Work out the finished part from the listing and answer in its coordinate system (mm). Face numbers are marked on the shaded views. A direction names the side the tool comes from. Coordinates: 2 decimals unless noted, no trailing zeros. Order: outer loops, then holes, each group sorted by start corner. A loop starts at its lowest first (then second) coordinate and runs counter-clockwise, first axis right, second up.
1. A tool of negligible diameter and unlimited length cuts with its end or side. For the marked faces 5, 6 and 7, from which of +Z, -Z, +X, -X, +Y, -Y can it reach the whole face along a straight path? Write none if from no direction.
2. The part is cut by section C-C, the plane x = -49. Give the vertices of the cut face in (y, z), then the cut area to 3 significant figures.
3. Find the intervals of material crossed by probe 1 along X at (y, z) = (-13, 17) (3 decimals); probe 2 along Y at (x, z) = (-31, 6.25); probe 3 along Y at (x, z) = (65, 6.5), in increasing order.
4. The part is cut by section A-A, the plane y = -11. Give the vertices of the cut face in (x, z) (3 decimals), then the cut area to 3 significant figures.
5. The part is cut by section D-D, the plane y = -4.5. Give the vertices of the cut face in (x, z), then the cut area to 3 significant figures.
6. Determine the mould class of the marked faces 1, 2, 3 and 4 for opening direction X: +X half, -X half, draft (parallel to the pull), parting line (faces both ways), or undercut.
7. Flat-ended cylindrical pins translate along their axes: pin 1 Ø5 at (y, z) = (-24, 6.5) entering from -X (3 decimals); pin 2 Ø9.5 at (y, z) = (-20, 13.5) entering from +X (3 decimals); pin 3 Ø8 at (x, y) = (44.5, -29) entering from -Z; pin 4 Ø1 at (x, z) = (57.5, 12.5) entering from +Y. Find the tip coordinate at first contact, or state that the pin passes through.
```python
from build123d import *

# Parameters (mm, degrees)
F0_W     = 25.4
F0_H     = 3.175
F1_DEPTH = 19.05


with BuildPart() as f1:
    # F0 (on Top) → F1 (new body)
    with BuildSketch(Plane.XY):
        with BuildLine():
            Line((-38.1, -1.5875), (-38.1, 1.5875))
            ThreePointArc((-38.1, 1.5875), (-44.835192, -1.202308), (-47.625, -7.9375))
            Line((-47.625, -7.9375), (-44.45, -7.9375))
            ThreePointArc((-44.45, -7.9375), (-42.590128, -3.447372), (-38.1, -1.5875))
        make_face()
        with BuildLine():
            Line((-44.45, -7.9375), (-47.625, -7.9375))
            ThreePointArc((-47.625, -7.9375), (-46.795096, -11.826065), (-44.45, -15.037016))
            Line((-44.45, -15.037016), (-44.45, -7.9375))
        make_face()
        with BuildLine():
            ThreePointArc((-44.45, -15.037016), (-46.795096, -11.826065), (-47.625, -7.9375))
            Line((-47.625, -7.9375), (-47.625, -30.1625))
            Line((-47.625, -30.1625), (-47.625, -33.3375))
            Line((-47.625, -33.3375), (-44.45, -33.3375))
            Line((-44.45, -33.3375), (-44.45, -15.037016))
        make_face()
        with Locations((-60.325, -31.75)):
            Rectangle(F0_W, F0_H)
        with BuildLine():
            ThreePointArc((-31.000484, -1.5875), (-34.211435, 0.757596), (-38.1, 1.5875))
            Line((-38.1, 1.5875), (-38.1, -1.5875))
            Line((-38.1, -1.5875), (-31.000484, -1.5875))
        make_face()
        with BuildLine():
            Line((0, 1.5875), (-38.1, 1.5875))
            ThreePointArc((-38.1, 1.5875), (-34.211435, 0.757596), (-31.000484, -1.5875))
            Line((-31.000484, -1.5875), (0, -1.5875))
            Line((0, -1.5875), (0, 1.5875))
        make_face()
        with BuildLine():
            Line((38.1, 1.5875), (0, 1.5875))
            Line((0, 1.5875), (0, -1.5875))
            Line((0, -1.5875), (31.000484, -1.5875))
            ThreePointArc((31.000484, -1.5875), (34.211435, 0.757596), (38.1, 1.5875))
        make_face()
        with BuildLine():
            Line((38.1, -1.5875), (38.1, 1.5875))
            ThreePointArc((38.1, 1.5875), (34.211435, 0.757596), (31.000484, -1.5875))
            Line((31.000484, -1.5875), (38.1, -1.5875))
        make_face()
        with BuildLine():
            ThreePointArc((47.625, -7.9375), (44.835192, -1.202308), (38.1, 1.5875))
            Line((38.1, 1.5875), (38.1, -1.5875))
            ThreePointArc((38.1, -1.5875), (42.590128, -3.447372), (44.45, -7.9375))
            Line((44.45, -7.9375), (47.625, -7.9375))
        make_face()
        with BuildLine():
            ThreePointArc((44.45, -15.037016), (46.795096, -11.826065), (47.625, -7.9375))
            Line((47.625, -7.9375), (44.45, -7.9375))
            Line((44.45, -7.9375), (44.45, -15.037016))
        make_face()
        with BuildLine():
            Line((47.625, -30.1625), (47.625, -7.9375))
            ThreePointArc((47.625, -7.9375), (46.795096, -11.826065), (44.45, -15.037016))
            Line((44.45, -15.037016), (44.45, -33.3375))
            Line((44.45, -33.3375), (47.625, -33.3375))
            Line((47.625, -33.3375), (47.625, -30.1625))
        make_face()
        with Locations((60.325, -31.75)):
            Rectangle(F0_W, F0_H)
    extrude(amount=F1_DEPTH)


solid = f1.part
```
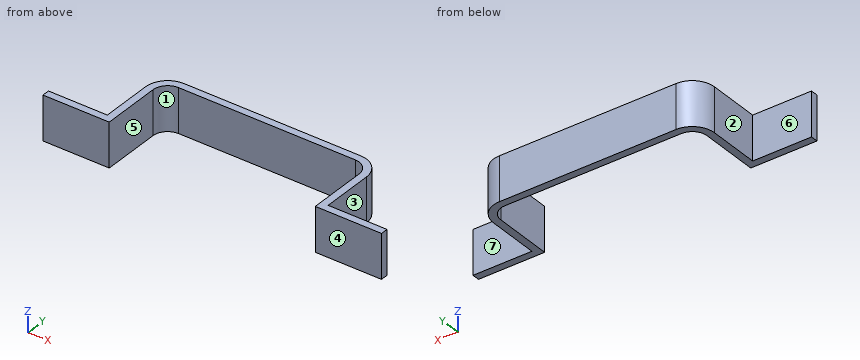
Geometry says:
1. face 5: +Z, -Z, -Y
1. face 6: +Z, -Z, -X, +Y
1. face 7: +Z, -Z, +X, +Y
2. outline: (-33.34, 0) - (-30.16, 0) - (-30.16, 19.05) - (-33.34, 19.05) - close
2. area: 60.5 mm2
3. probe 1: x = -47.625 to -44.45, 44.45 to 47.625
3. probe 2: y = -1.59 to 1.59
3. probe 3: y = -33.34 to -30.16
4. outline: (-47.625, 0) - (-44.45, 0) - (-44.45, 19.05) - (-47.625, 19.05) - close; (44.45, 0) - (47.625, 0) - (47.625, 19.05) - (44.45, 19.05) - close
4. area: 121 mm2
5. outline: (-46.98, 0) - (-43.44, 0) - (-43.44, 19.05) - (-46.98, 19.05) - close; (43.44, 0) - (46.98, 0) - (46.98, 19.05) - (43.44, 19.05) - close
5. area: 135 mm2
6. face 1: undercut
6. face 2: -X half
6. face 3: +X half
6. face 4: draft
7. pin 1: stops at x = -47.625
7. pin 2: stops at x = 47.625
7. pin 3: stops at z = 0
7. pin 4: stops at y = -30.16
